Verification items for the finished model (mm, model axes). A direction names the side the tool comes from. Coordinates: 2 decimals unless noted, no trailing zeros. Order: outer loops, then holes, each group sorted by start corner. A loop starts at its lowest first (then second) coordinate and runs counter-clockwise, first axis right, second up.
Q1. Cross-section at B-B, the plane z = 0. Record the boundary of the cut face in (x, y) (3 decimals), and give its area (3 significant figures).
Q2. Cross-section at A-A, the plane x = 0. Record the boundary of the cut face in (y, z) (3 decimals).
Q3. Thickness scan on line 1 (Z direction, x = -33, y = 2.15); line 2 (X direction, y = 2, z = 32.5); line 3 (X direction, y = 0.45, z = 33). Record the ranges inside material, lowest first.
Q4. Cross-section at D-D, the plane y = 1.1. Count the separate pieces of the cut face and the enclosed holes in it, and give its area (3 significant figures).
Q5. Cross-section at C-C, the plane z = 34. Record the boundary of the cut face in (x, y) (3 decimals).
Q6. Draft check along Z on faces 1 (the flat face through (-18.07, 1.57, -10.5)), 2 (the cylindrical face through (-39.14, 1.61, 39.1)), 3 (the cylindrical face through (-15.319, 1.565, 13.917)), 4 (the flat face through (-40, 2, 1)). Enter one of: pulls with the +Z half, pulls with the -Z half, needs draft (parallel to the pull), parting line crosses it, or undercut.
Q7. Set-up check for faces 5 (the flat face through (-14.11, 1.57, -8.16)), 6 (the flat face through (-9, 3.175, -9)): record each of +Z, -Z, +X, -X, +Y, -Y from which the full face is reachable in a straight line by a thin tool's end or side.
from build123d import *

# Parameters (mm, degrees)
SKETCH1_W           = 80
SKETCH1_H           = 80
SKETCH1_R           = 11.25
SKETCH1_R_2         = 2.15
SKETCH1_R_3         = 4.5
BOSS_EXTRUDE1_DEPTH = 3.175
FILLET1_R           = 3
FILLET2_R           = 1


with BuildPart() as part:
    # Sketch1 → Boss-Extrude1 (new body)
    with BuildSketch(Plane(origin=(0, 0, 0), x_dir=(1, 0, 0), z_dir=(0, 1, 0))):
        Rectangle(SKETCH1_W, SKETCH1_H)
        with Locations(Location((0, 0, 0), (0, 0, 270))):
            Circle(SKETCH1_R, mode=Mode.SUBTRACT)
        with Locations(Location((0, 29, 0), (0, 0, 270))):
            Circle(SKETCH1_R_2, mode=Mode.SUBTRACT)
        with Locations(Location((25.11473671, -14.5, 0), (0, 0, 270))):
            Circle(SKETCH1_R_2, mode=Mode.SUBTRACT)
        with Locations(Location((-25.11473671, -14.5, 0), (0, 0, 270))):
            Circle(SKETCH1_R_2, mode=Mode.SUBTRACT)
        with Locations(Location((-34, -34, 0), (0, 0, 270))):
            Circle(SKETCH1_R_2, mode=Mode.SUBTRACT)
        with Locations(Location((34, -34, 0), (0, 0, 90))):
            Circle(SKETCH1_R_2, mode=Mode.SUBTRACT)
        with Locations(Location((33.43865922, 33.896147379, 0), (0, 0, 270))):
            Circle(SKETCH1_R_2, mode=Mode.SUBTRACT)
        with Locations(Location((-34.552045293, 32.77182544, 0), (0, 0, 90))):
            Circle(SKETCH1_R_2, mode=Mode.SUBTRACT)
        with Locations(Location((-16.670989023, -9.625, 0), (0, 0, 270))):
            Circle(SKETCH1_R_3, mode=Mode.SUBTRACT)
        Polygon((-19.626238937, 7.781840133), (-15.635110011, 5.494726254), (-12.552478261, 10.874073937), (-16.543607188, 13.161187816), align=None, mode=Mode.SUBTRACT)
    extrude(amount=BOSS_EXTRUDE1_DEPTH)

    # Fillet1
    fillet1_edges = [part.edges().sort_by_distance(p)[0] for p in [
        (40, 1.5875, 40),
        (-40, 1.5875, 40),
        (-40, 1.5875, -40),
        (40, 1.5875, -40),
    ]]
    fillet(fillet1_edges, radius=FILLET1_R)

    # Fillet2
    fillet2_edges = [part.edges().sort_by_distance(p)[0] for p in [
        (-16.543607188, 1.5875, -13.161187816),
        (-19.626238937, 1.5875, -7.781840133),
        (-15.635110011, 1.5875, -5.494726254),
        (-12.552478261, 1.5875, -10.874073937),
    ]]
    fillet(fillet2_edges, radius=FILLET2_R)


solid = part.part
Check values:
1. outline: (-40, 0) - (-11.25, 0) - (-11.25, 3.175) - (-40, 3.175) - close; (11.25, 0) - (40, 0) - (40, 3.175) - (11.25, 3.175) - close
1. area: 183 mm2
2. outline: (0, -40) - (3.175, -40) - (3.175, -31.15) - (0, -31.15) - close; (0, -26.85) - (3.175, -26.85) - (3.175, -11.25) - (0, -11.25) - close; (0, 11.25) - (3.175, 11.25) - (3.175, 40) - (0, 40) - close
3. line 1: z = -40 to -34.26, -31.28 to 32.1, 35.9 to 40
3. line 2: x = -40 to -35.54, -32.46 to 32.46, 35.54 to 40
3. line 3: x = -40 to -35.9, -32.1 to 32.1, 35.9 to 40
4. separate pieces: 1
4. enclosed holes: 10
4. area: 5,800 mm2
5. outline: (-40, 0) - (-36.15, 0) - (-36.15, 3.175) - (-40, 3.175) - close; (-31.85, 0) - (31.85, 0) - (31.85, 3.175) - (-31.85, 3.175) - close; (36.15, 0) - (40, 0) - (40, 3.175) - (36.15, 3.175) - close
6. face 1: undercut
6. face 2: pulls with the +Z half
6. face 3: undercut
6. face 4: needs draft
7. face 5: +Y, -Y
7. face 6: +Z, -Z, +X, -X, +Y
